Geometry: see drawing. Coordinates: mm, zero at the bounding-box minimum. Give positions to 0.01 mm unless a question says otherwise; leave off trailing zeros. Write each loop counter-clockwise with the first axis right and the second up, starting at its lowest first coordinate (ties: lowest second). Pieces come first, ordered by that corner, then holes. Notation, with made-up numbers: (68.5, 87) - (96.5, 87) arc R27 cw to (96.5, 111) - close; hole circle Ø2 at (1, -22.5). An arc over 180 degrees is marked (long way). Return JSON: item names as keys, results as strings.
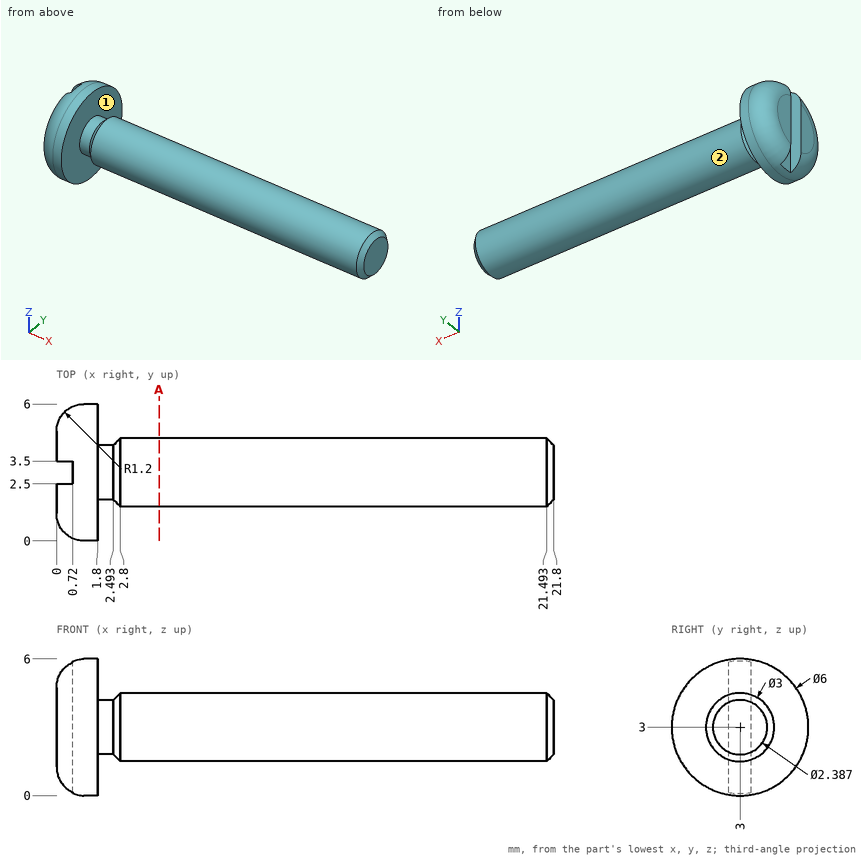
Q1. Section query A-A, the plane x = 4.5. Return the cut outline in (y, z).
Answer key:
{"outline": "circle Ø3 at (3, 3)"}
Q2. Pin query (flat end, axial travel): P1, Ø2, axis at x = 5, z = 2, coming from the -Y side; P2, Ø0.8, axis at y = 3, z = 4, coming from the -X side; P3, Ø2, axis at y = 2, z = 2, coming from the +X side; P4, Ø0.6, axis at x = 0, z = 4.5, coming from the -Y side. Return the tip coordinate at first contact, or that it passes through.
Answer key:
{"P1": "stops at y = 1.5", "P2": "stops at x = 0.72", "P3": "stops at x = 21.8", "P4": "stops at y = 0.84"}
Q3. Material intervals for probe 1 along X at (y, z) = (4.25, 5); probe 2 along X at (y, z) = (2.25, 1.5); probe 3 along Z at (x, y) = (21, 1.75), sorted ascending. Write a range as [from, to].
Answer key:
{"probe 1": "x = [0.14, 1.8]", "probe 2": "x = [0, 1.8]", "probe 3": "z = [2.17, 3.83]"}
Q4. Mould query, pull axis Y, two halves, no side actions, for the marked faces 1 and 2. Classes: pulls with the +Y half, pulls with the -Y half, needs draft (parallel to the pull), parting line crosses it, or undercut.
Answer key:
{"face 1": "needs draft", "face 2": "parting line crosses it"}
